Build history of the part. All positions in model axes, mm. Give positions to 0.01 mm unless a question says otherwise; leave off trailing zeros. Use a Markdown table: item, result. Add a question column.
(1) Wall check: line 1 (Y direction, x = -41, z = 5.25); line 2 (X direction, y = -4, z = 5.5); line 3 (X direction, y = 3.75, z = 2.25). Give the ranges that are in metal, low to high.
(2) Mould opens along X. For faces 1 (the face through (36, -1.16, 3)), 2 (the face through (36, 0.161, 3)), 3 (the face through (0, 0, 0)), 4 (the face through (47.945, -1, 3)) say: +X half, -X half, draft (parallel to the pull), parting line (faces both ways), or undercut.
(3) Slice it at A-A (z = 4.5). Count the separate pieces of the cut face and the enclosed holes in it, then the cut area to 3 significant figures.
(4) Flat gauge pin, fed straight in: pin 1 (1 mm diameter, centred on x = -28.25, y = -0.5, fed in from +Z). Where does the tip first touch, or does it go through?
from build123d import *

# Parameters (mm, degrees)
BOSS_EXTRUDE3_DEPTH = 6.35
CUT_EXTRUDE2_DEPTH  = 25.4


with BuildPart() as part:
    # Sketch1 → Boss-Extrude3 (new body)
    # profile 1 of 2: a face of its own
    with BuildSketch(Plane.XY):
        with BuildLine():
            ThreePointArc((-40.954752736, 5.850678962), (-47.304752736, -0.499321038), (-40.954752736, -6.849321038))
            Line((-40.954752736, -6.849321038), (47.945247264, -6.849321038))
            Line((47.945247264, -6.849321038), (47.945247264, 5.850678962))
            Line((47.945247264, 5.850678962), (-40.954752736, 5.850678962))
        make_face()
        with BuildLine():
            ThreePointArc((-40.319752736, -0.499321038), (-40.954490658, -1.134320984), (-41.589752519, -0.499845193))
            ThreePointArc((-41.589752519, -0.499845193), (-40.955276891, 0.135678746), (-40.319752952, -0.498796882))
            ThreePointArc((-40.319752952, -0.498796882), (-40.31975279, -0.49905896), (-40.319752736, -0.499321038))
        make_face(mode=Mode.SUBTRACT)
        with BuildLine():
            Line((-37.144752749, -0.499189999), (-37.144752736, -0.499321038))
            ThreePointArc((-37.144752736, -0.499321038), (-38.414752732, -0.499386557), (-37.144752749, -0.499189999))
        make_face(mode=Mode.SUBTRACT)
        with BuildLine():
            ThreePointArc((-33.969752736, -0.499321038), (-34.604752736, -1.134321038), (-35.239752736, -0.499321038))
            ThreePointArc((-35.239752736, -0.499321038), (-34.604752736, 0.135678962), (-33.969752736, -0.499321038))
        make_face(mode=Mode.SUBTRACT)
        with BuildLine():
            ThreePointArc((-30.794752736, -0.499321038), (-31.429752736, -1.134321038), (-32.064752736, -0.499321038))
            ThreePointArc((-32.064752736, -0.499321038), (-31.429752736, 0.135678962), (-30.794752736, -0.499321038))
        make_face(mode=Mode.SUBTRACT)
        with BuildLine():
            ThreePointArc((-27.619752736, -0.499321038), (-28.254752736, -1.134321038), (-28.889752736, -0.499321038))
            ThreePointArc((-28.889752736, -0.499321038), (-28.254752736, 0.135678962), (-27.619752736, -0.499321038))
        make_face(mode=Mode.SUBTRACT)
        with BuildLine():
            ThreePointArc((-24.444752736, -0.499321038), (-25.079752736, -1.134321038), (-25.714752736, -0.499321038))
            ThreePointArc((-25.714752736, -0.499321038), (-25.079752736, 0.135678962), (-24.444752736, -0.499321038))
        make_face(mode=Mode.SUBTRACT)
        with BuildLine():
            ThreePointArc((32.070247264, -0.499321038), (32.705247264, 0.135678962), (33.340247264, -0.499321038))
            ThreePointArc((33.340247264, -0.499321038), (32.705247264, -1.134321038), (32.070247264, -0.499321038))
        make_face(mode=Mode.SUBTRACT)
        with BuildLine():
            ThreePointArc((35.245247264, -0.499321038), (35.880247264, 0.135678962), (36.515247264, -0.499321038))
            ThreePointArc((36.515247264, -0.499321038), (35.880247264, -1.134321038), (35.245247264, -0.499321038))
        make_face(mode=Mode.SUBTRACT)
        with BuildLine():
            ThreePointArc((38.420247264, -0.499321038), (39.055247264, 0.135678962), (39.690247264, -0.499321038))
            ThreePointArc((39.690247264, -0.499321038), (39.055247264, -1.134321038), (38.420247264, -0.499321038))
        make_face(mode=Mode.SUBTRACT)
    # profile 2 of 2: a face of its own
    with BuildSketch(Plane.XY):
        with BuildLine():
            ThreePointArc((-40.954752736, 5.850678962), (-47.304752736, -0.499321038), (-40.954752736, -6.849321038))
            Line((-40.954752736, -6.849321038), (47.945247264, -6.849321038))
            Line((47.945247264, -6.849321038), (47.945247264, 5.850678962))
            Line((47.945247264, 5.850678962), (-40.954752736, 5.850678962))
        make_face()
        with BuildLine():
            ThreePointArc((-40.319752736, -0.499321038), (-40.954490658, -1.134320984), (-41.589752519, -0.499845193))
            ThreePointArc((-41.589752519, -0.499845193), (-40.955276891, 0.135678746), (-40.319752952, -0.498796882))
            ThreePointArc((-40.319752952, -0.498796882), (-40.31975279, -0.49905896), (-40.319752736, -0.499321038))
        make_face(mode=Mode.SUBTRACT)
        with BuildLine():
            Line((-37.144752749, -0.499189999), (-37.144752736, -0.499321038))
            ThreePointArc((-37.144752736, -0.499321038), (-38.414752732, -0.499386557), (-37.144752749, -0.499189999))
        make_face(mode=Mode.SUBTRACT)
        with BuildLine():
            ThreePointArc((-33.969752736, -0.499321038), (-34.604752736, -1.134321038), (-35.239752736, -0.499321038))
            ThreePointArc((-35.239752736, -0.499321038), (-34.604752736, 0.135678962), (-33.969752736, -0.499321038))
        make_face(mode=Mode.SUBTRACT)
        with BuildLine():
            ThreePointArc((-30.794752736, -0.499321038), (-31.429752736, -1.134321038), (-32.064752736, -0.499321038))
            ThreePointArc((-32.064752736, -0.499321038), (-31.429752736, 0.135678962), (-30.794752736, -0.499321038))
        make_face(mode=Mode.SUBTRACT)
        with BuildLine():
            ThreePointArc((-27.619752736, -0.499321038), (-28.254752736, -1.134321038), (-28.889752736, -0.499321038))
            ThreePointArc((-28.889752736, -0.499321038), (-28.254752736, 0.135678962), (-27.619752736, -0.499321038))
        make_face(mode=Mode.SUBTRACT)
        with BuildLine():
            ThreePointArc((-24.444752736, -0.499321038), (-25.079752736, -1.134321038), (-25.714752736, -0.499321038))
            ThreePointArc((-25.714752736, -0.499321038), (-25.079752736, 0.135678962), (-24.444752736, -0.499321038))
        make_face(mode=Mode.SUBTRACT)
        with BuildLine():
            ThreePointArc((32.070247264, -0.499321038), (32.705247264, 0.135678962), (33.340247264, -0.499321038))
            ThreePointArc((33.340247264, -0.499321038), (32.705247264, -1.134321038), (32.070247264, -0.499321038))
        make_face(mode=Mode.SUBTRACT)
        with BuildLine():
            ThreePointArc((35.245247264, -0.499321038), (35.880247264, 0.135678962), (36.515247264, -0.499321038))
            ThreePointArc((36.515247264, -0.499321038), (35.880247264, -1.134321038), (35.245247264, -0.499321038))
        make_face(mode=Mode.SUBTRACT)
        with BuildLine():
            ThreePointArc((38.420247264, -0.499321038), (39.055247264, 0.135678962), (39.690247264, -0.499321038))
            ThreePointArc((39.690247264, -0.499321038), (39.055247264, -1.134321038), (38.420247264, -0.499321038))
        make_face(mode=Mode.SUBTRACT)
    extrude(amount=BOSS_EXTRUDE3_DEPTH)

    # Sketch2 → Cut-Extrude2 (cut)
    with BuildSketch(Plane.XY.offset(6.35)):
        with BuildLine():
            Line((32.705247264, -1.159721038), (39.055247264, -1.159721038))
            ThreePointArc((39.055247264, -1.159721038), (39.715647264, -0.499321038), (39.055247264, 0.161078962))
            Line((39.055247264, 0.161078962), (32.705247264, 0.161078962))
            ThreePointArc((32.705247264, 0.161078962), (32.044847264, -0.499321038), (32.705247264, -1.159721038))
        make_face()
    extrude(amount=-CUT_EXTRUDE2_DEPTH, mode=Mode.SUBTRACT)


solid = part.part
Solution:
| question | item | result |
|---|---|---|
| 1 | line 1 | -6.85 to -1.13, 0.13 to 5.85 |
| 1 | line 2 | -46.25 to 47.95 |
| 1 | line 3 | -45.67 to 47.95 |
| 2 | face 1 | undercut |
| 2 | face 2 | undercut |
| 2 | face 3 | draft |
| 2 | face 4 | +X half |
| 3 | separate pieces | 1 |
| 3 | enclosed holes | 7 |
| 3 | area | 1,180 mm2 |
| 4 | pin 1 | through |
